Solid Edge part; units mm, degrees
sketch "Sketch1" plane through (0, 0, 0) normal (0, 0, 1) x (1, 0, 0)
  line L0 (-50.7701, 18.3701) -> (50.7701, 18.3701)
  line L1 (50.7701, 18.3701) -> (50.7701, -18.3701)
  line L2 (50.7701, -18.3701) -> (-50.7701, -18.3701)
  line L3 (-50.7701, -18.3701) -> (-50.7701, 18.3701)
  dimension "D1" = 50.7701
  dimension "D2" = 50.7701
extrude "Protrusion1" add sketch "Sketch1" along normal blind 2
sketch "Sketch2" plane through (0, 0, 2) normal (0, 0, 1) x (0, -1, 0)
  line L0 (-14.6299, 39.6399) -> (18.3701, 39.6399)
  line L1 (18.3701, -0.5383) -> (18.3701, 39.6399)
  line L2 (18.3701, -0.5383) -> (12.7975, -46.7701)
  line L3 (12.7975, -46.7701) -> (12.7975, -50.7701)
  line L4 (12.7975, -50.7701) -> (-9.1299, -50.7701)
  line L5 (-9.0573, -46.7701) -> (-9.1299, -50.7701)
  line L6 (-9.0573, -46.7701) -> (-14.6299, -0.5383)
  line L7 (-14.6299, -0.5383) -> (-14.6299, 39.6399)
extrude "Extrusionsausschnitt_1" cut sketch "Sketch2" against normal blind 130.0765 flip side to cut
hole "Bohrung_1" at (-10.7701, -1.8701, 2) direction (0, 0, -1) diameter 3.5 end up to next countersink diameter 6.94 countersink angle 90
hole "Hole1" at (-30.7701, -1.8701, 2) direction (0, 0, -1) diameter 3.5 end up to next countersink diameter 6.94 countersink angle 90
hole "Hole2" at (32.2299, -1.8701, 2) direction (0, 0, -1) diameter 3.5 end up to next countersink diameter 6.94 countersink angle 90
fillet "Verrundung_1" radius 5 2 edges at (39.6399, -18.3701, 1) (39.6399, 14.6299, 1)
Can you work these out from the model? Positions are in its coordinate system, mm. A direction names the side the tool comes from. Coordinates: 2 decimals unless noted, no trailing zeros. Order: outer loops, then holes, each group sorted by start corner. A loop starts at its lowest first (then second) coordinate and runs counter-clockwise, first axis right, second up.
1. For faces 1 (the face through (-49, -12.798, 1)), 2 (the face through (17, -18.37, 1)), which set-ups out of +Z, -Z, +X, -X, +Y, -Y let a thin tool reach every point of the face, with its end or its side?
2. If we section it at D-D (y = 11.5): Please give me the cut outline in (x, z).
3. If we section it at A-A (z = 1.3): Please give me the cut outline in (x, y), then the cut area to 3 significant figures.
4. Thinking about a two-plate mould opening in X: for faces 3 (the face through (38.14, 13.2, 0.99)), 4 (the face through (-32.584, -1.467, 0.388)), 5 (the face through (17, 14.63, 1)), which applies, +X half, -X half, draft (parallel to the pull), parting line (faces both ways), or undercut?
5. I need wall thicknesses on line 1 (X direction, y = -2, z = 0.3); line 2 (X direction, y = -2, z = 1.2); line 3 (Y direction, x = 33.5, z = 0.3). Which ranges of each line are inside material? Lowest first, please.
6. If we section it at B-B (y = -2.5): Give the number of separate pieces and of enclosed holes in the cut face, then the cut area to 3 significant figures.
7. If we section it at C-C (x = -41): Please give me the cut outline in (y, z).
8. I'm going to push flat-ended pins straight in: pin 1 (6 mm diameter, centred on x = -28, y = 4.5, fed in from -Z); pin 2 (4 mm diameter, centred on x = -30.77, y = -1.87, fed in from +Z). Where does each tip first touch, or does it pass through?
Entries:
1. face 1: +Z, -Z, -X, -Y
1. face 2: +Z, -Z, +X, -X, -Y
2. outline: (-26.5, 0) - (39.28, 0) - (39.28, 2) - (-26.5, 2) - close
3. outline: (-50.77, -12.8) - (-46.77, -12.8) - (-0.54, -18.37) - (34.64, -18.37) arc R5 ccw to (39.64, -13.37) - (39.64, 9.63) arc R5 ccw to (34.64, 14.63) - (-0.54, 14.63) - (-46.77, 9.06) - (-50.77, 9.13) - close; hole circle Ø5.54 at (-30.77, -1.87); hole circle Ø5.54 at (-10.77, -1.87); hole circle Ø5.54 at (32.23, -1.87)
3. area: 2,600 mm2
4. face 3: +X half
4. face 4: undercut
4. face 5: draft
5. line 1: x = -50.77 to -32.54, -29 to -12.54, -9 to 30.46, 34 to 39.64
5. line 2: x = -50.77 to -33.44, -28.1 to -13.44, -8.1 to 29.56, 34.9 to 39.64
5. line 3: y = -18.37 to -3.1, -0.64 to 14.63
6. separate pieces: 4
6. enclosed holes: 0
6. area: 152 mm2
7. outline: (-13.49, 0) - (9.75, 0) - (9.75, 2) - (-13.49, 2) - close
8. pin 1: stops at z = 0
8. pin 2: stops at z = 0.53
